from build123d import *

# Parameters (mm, degrees)
SKETCH1_W                      = 100
SKETCH1_H                      = 30
BOSS_EXTRUDE1_DEPTH            = 50
SHELL1_T                       = -3
CUT_EXTRUDE1_REACH             = 116.495
SKETCH2_W                      = 22.5
SKETCH2_H                      = 12.2
F_2_2_2_2_DIAMETER_HOLE1_D     = 2.2
F_2_2_2_2_DIAMETER_HOLE1_DEPTH = 3
CUT_EXTRUDE2_REACH             = 116.495
SKETCH5_W                      = 15
SKETCH5_H                      = 3
CUT_EXTRUDE3_REACH             = 117.758
SKETCH6_W                      = 8.2
SKETCH6_H                      = 8.2
F_2_05_2_05_DIAMETER_HOLE1_D   = 2.05


with BuildPart() as part:
    # Sketch1 → Boss-Extrude1 (new body)
    with BuildSketch(Plane(origin=(0, 0, 0), x_dir=(1, 0, 0), z_dir=(0, 1, 0))):
        with Locations((50, 15)):
            Rectangle(SKETCH1_W, SKETCH1_H)
    extrude(amount=BOSS_EXTRUDE1_DEPTH)

    # Shell1
    shell1_openings = [part.faces().sort_by_distance(p)[0] for p in [
        (50, 25, -30),
    ]]
    offset(amount=SHELL1_T, openings=shell1_openings, kind=Kind.INTERSECTION)

    # Sketch2 → Cut-Extrude1 (cut, up to next)
    with BuildSketch(Plane(origin=(0, 3, 0), x_dir=(1, 0, 0), z_dir=(0, 1, 0)), mode=Mode.PRIVATE) as cut_extrude1_sk1:
        with Locations((54.15, 12)):
            Rectangle(SKETCH2_W, SKETCH2_H)
    cut_extrude1_tool1 = extrude(cut_extrude1_sk1.sketch, amount=-CUT_EXTRUDE1_REACH, mode=Mode.PRIVATE) & part.part
    add(cut_extrude1_tool1.solids().sort_by_distance((54.15, 3, -12))[0], mode=Mode.SUBTRACT)

    # Ø2.2 (2.2) Diameter Hole1
    with Locations(Plane(origin=(0, 3, 0), x_dir=(1, 0, 0), z_dir=(0, 1, 0))):
        with Locations((68.055, 12), (40.245, 12)):
            Hole(F_2_2_2_2_DIAMETER_HOLE1_D / 2, depth=F_2_2_2_2_DIAMETER_HOLE1_DEPTH)

    # Sketch5 → Cut-Extrude2 (cut, up to next)
    with BuildSketch(Plane(origin=(0, 3, 0), x_dir=(1, 0, 0), z_dir=(0, 1, 0)), mode=Mode.PRIVATE) as cut_extrude2_sk1:
        with Locations((49, 24.5)):
            Rectangle(SKETCH5_W, SKETCH5_H)
    cut_extrude2_tool1 = extrude(cut_extrude2_sk1.sketch, amount=-CUT_EXTRUDE2_REACH, mode=Mode.PRIVATE) & part.part
    add(cut_extrude2_tool1.solids().sort_by_distance((49, 3, -24.5))[0], mode=Mode.SUBTRACT)

    # Sketch6 → Cut-Extrude3 (cut, up to next)
    with BuildSketch(Plane.XY, mode=Mode.PRIVATE) as cut_extrude3_sk1:
        with Locations((80.1, 25)):
            Rectangle(SKETCH6_W, SKETCH6_H)
    cut_extrude3_tool1 = extrude(cut_extrude3_sk1.sketch, amount=-CUT_EXTRUDE3_REACH, mode=Mode.PRIVATE) & part.part
    # Sketch6 → Cut-Extrude3 (cut, up to next)
    with BuildSketch(Plane.XY, mode=Mode.PRIVATE) as cut_extrude3_sk2:
        with Locations((21.9, 25)):
            Rectangle(SKETCH6_W, SKETCH6_H)
    cut_extrude3_tool2 = extrude(cut_extrude3_sk2.sketch, amount=-CUT_EXTRUDE3_REACH, mode=Mode.PRIVATE) & part.part
    add(cut_extrude3_tool1.solids().sort_by_distance((80.1, 25, 0))[0], mode=Mode.SUBTRACT)
    add(cut_extrude3_tool2.solids().sort_by_distance((21.9, 25, 0))[0], mode=Mode.SUBTRACT)

    # Ø2.05 (2.05) Diameter Hole1 (through all)
    with Locations(Plane(origin=(0, 0, -3), x_dir=(-1, 0, 0), z_dir=(0, 0, -1))):
        with Locations((-90.6, 25), (-69.6, 25), (-32.4, 25), (-11.4, 25)):
            Hole(F_2_05_2_05_DIAMETER_HOLE1_D / 2)


solid = part.part
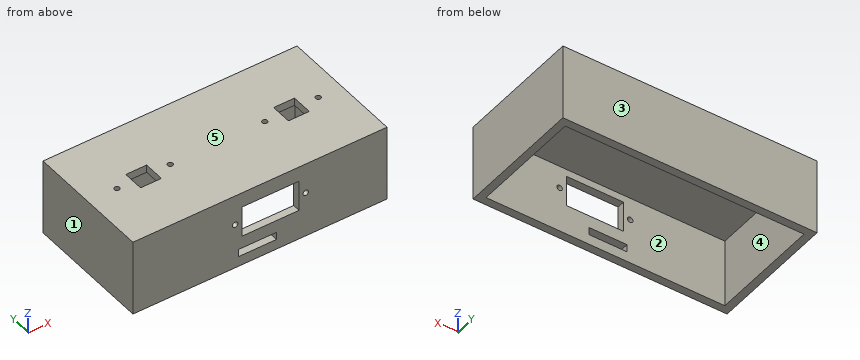
The listing builds one solid part. Answer for the finished solid, in the listing's coordinates (mm). Face numbers are marked on the shaded views. A direction names the side the tool comes from. Give positions to 0.01 mm unless a question says otherwise; leave off trailing zeros. Write each loop counter-clockwise with the first axis right and the second up, starting at its lowest first coordinate (ties: lowest second). Pieces come first, ordered by that corner, then holes.
Item 1: Section D-D, the plane x = 52.5 is taken. Write down the section's boundary in (y, z).
Item 2: Find the intervals of material crossed by line 1 along X through (y, z) = (24.5, -13.25); line 2 along Y through (x, z) = (32.4, -1.15) (3 decimals); line 3 along Y through (x, z) = (62, -22), in increasing order.
Item 3: Section C-C, the plane z = -20.25 is taken. Write down the section's boundary in (x, y), plus the area to 3 significant figures.
Item 4: Flat-ended cylindrical pins translate along their axes: P1, Ø3, axis at x = 31, y = 39, coming from the -Z side; P2, Ø1.8, axis at x = 11.4, y = 25, coming from the +Z side. Find the tip coordinate at first contact, or state that the pin passes through.
Item 5: Section A-A, the plane y = 25 is taken. Count the separate pieces of the cut face and the enclosed holes in it, plus the area to 3 significant figures.
Item 6: Section B-B, the plane x = 90.6 is taken. Write down the section's boundary in (y, z) (3 decimals), plus the area to 3 significant figures.
Item 7: Determine the mould class of the marked faces 3, 4 and 5 for opening direction Y: released by +Y, released by -Y, zero draft, split by the parting line, or undercut.
Item 8: Which of the six approach directions +Z, -Z, +X, -X, +Y, -Y give full straight-line access (tool end or side, diameter ignored) to the marked faces 1 and 2?
Completed:
1. outline: (0, -30) - (3, -30) - (3, -26) - (0, -26) - close; (0, -23) - (3, -23) - (3, -18.1) - (0, -18.1) - close; (0, -5.9) - (3, -5.9) - (3, -3) - (47, -3) - (47, -30) - (50, -30) - (50, 0) - (0, 0) - close
2. line 1: x = 0 to 3, 97 to 100
2. line 2: y = 0 to 23.975, 26.025 to 50
2. line 3: y = 0 to 3, 47 to 50
3. outline: (0, 0) - (100, 0) - (100, 50) - (0, 50) - close; hole (3, 3) - (97, 3) - (97, 47) - (3, 47) - close
3. area: 864 mm2
4. P1: stops at z = -3
4. P2: passes through
5. separate pieces: 7
5. enclosed holes: 0
5. area: 388 mm2
6. outline: (0, -30) - (3, -30) - (3, -3) - (23.975, -3) - (23.975, 0) - (0, 0) - close; (26.025, -3) - (47, -3) - (47, -30) - (50, -30) - (50, 0) - (26.025, 0) - close
6. area: 306 mm2
7. face 3: released by +Y
7. face 4: undercut
7. face 5: zero draft
8. face 1: +Z, -Z, -X, +Y, -Y
8. face 2: -Z
